Build history of the part. All positions in model axes, mm. A direction names the side the tool comes from. Give positions to 0.01 mm unless a question says otherwise; leave off trailing zeros. Loops run counter-clockwise (first coordinate to the right, second up) from the corner with the lowest first, then second, coordinate; pieces in that order, holes last.
1) Band-saw the part on B-B on z = 6.75. List the corners of the cut face in (x, y).
2) Wall check: line 1 (Y direction, x = 18.35, z = 4.25); line 2 (X direction, y = -12, z = 4); line 3 (X direction, y = -4.5, z = 3). Give the ranges that are in metal, low to high.
3) Flat gauge pins, fed straight in: P1, Ø1.1, axis at x = 24, y = 8, coming from the -Z side; P2, Ø1.1, axis at x = 26.5, y = 0, coming from the +Z side; P3, Ø4, axis at x = 26.5, z = 2.5, coming from the +Y side. Where does each tip first touch, or does it go through?
4) Two-plate mould, pull along Y, no slides. Class faces 1 (the flat face through (25, -9, 4)), 2 (the flat face through (25, -3, 6.15)): +Y half, -Y half, draft (parallel to the pull), parting line (faces both ways), or undercut.
5) 3-axis set-ups, long thin cutter, end or side, ignore diameter. For faces 3 (the cylindrical face through (-25.05, -12.44, 3.11)), 4 (the cylindrical face through (17.05, -12.04, 3.7)), 5 (the flat face through (25, -6.833, 4)), 6 (the flat face through (25, 8, 6.15)), 7 (the flat face through (0, 0, 0)): which of +Z, -Z, +X, -X, +Y, -Y reach the whole face in a straight line?
6) Band-saw the part on C-C on z = 3.65. State how many separate pieces and enclosed holes the cut face has, then the cut area to 3 significant figures.
7) Band-saw the part on A-A on x = 18.35. List the corners of the cut face in (y, z).
```python
from build123d import *

# Parameters (mm, degrees)
SKETCH1_W           = 42.5
SKETCH1_H           = 30
BOSS_EXTRUDE1_DEPTH = 7.3
CUT_EXTRUDE1_REACH  = 9.3
SKETCH2_R           = 1.3
SKETCH3_R           = 2.5
BOSS_EXTRUDE2_DEPTH = 7.7
SKETCH4_W           = 5
SKETCH4_H           = 1
BOSS_EXTRUDE3_DEPTH = 7.5


with BuildPart() as part:
    # Sketch1 → Boss-Extrude1 (new body)
    with BuildSketch(Plane.XY):
        Rectangle(SKETCH1_W, SKETCH1_H)
    extrude(amount=BOSS_EXTRUDE1_DEPTH)

    # Sketch2 → Cut-Extrude1 (cut, up to next)
    with BuildSketch(Plane.XY.offset(7.3), mode=Mode.PRIVATE) as cut_extrude1_sk1:
        with Locations((18.35, -12.1)):
            Circle(SKETCH2_R)
    cut_extrude1_tool1 = extrude(cut_extrude1_sk1.sketch, amount=-CUT_EXTRUDE1_REACH, mode=Mode.PRIVATE) & part.part
    add(cut_extrude1_tool1.solids().sort_by_distance((18.35, -12.1, 7.3))[0], mode=Mode.SUBTRACT)
    # Sketch2 → Cut-Extrude1 (cut, up to next)
    with BuildSketch(Plane.XY.offset(7.3), mode=Mode.PRIVATE) as cut_extrude1_sk2:
        with Locations((18.35, 12.1)):
            Circle(SKETCH2_R)
    cut_extrude1_tool2 = extrude(cut_extrude1_sk2.sketch, amount=-CUT_EXTRUDE1_REACH, mode=Mode.PRIVATE) & part.part
    add(cut_extrude1_tool2.solids().sort_by_distance((18.35, 12.1, 7.3))[0], mode=Mode.SUBTRACT)
    # Sketch2 → Cut-Extrude1 (cut, up to next)
    with BuildSketch(Plane.XY.offset(7.3), mode=Mode.PRIVATE) as cut_extrude1_sk3:
        with Locations((-18.95, 0)):
            Circle(SKETCH2_R)
    cut_extrude1_tool3 = extrude(cut_extrude1_sk3.sketch, amount=-CUT_EXTRUDE1_REACH, mode=Mode.PRIVATE) & part.part
    add(cut_extrude1_tool3.solids().sort_by_distance((-18.95, 0, 7.3))[0], mode=Mode.SUBTRACT)

    # Sketch3 → Boss-Extrude2 (add)
    with BuildSketch(Plane.ZY.offset(21.25)):
        with Locations((3.65, 10)):
            Circle(SKETCH3_R)
        with Locations((3.65, -10)):
            Circle(SKETCH3_R)
    extrude(amount=BOSS_EXTRUDE2_DEPTH)

    # Sketch4 → Boss-Extrude3 (add)
    with BuildSketch(Plane(origin=(21.25, 0, 0), x_dir=(0, 0, -1), z_dir=(1, 0, 0))):
        with Locations((-3.65, 9.5)):
            Rectangle(SKETCH4_W, SKETCH4_H)
        with Locations((-3.65, 7.916666667)):
            Rectangle(SKETCH4_W, SKETCH4_H)
        with Locations((-3.65, 6.333333333)):
            Rectangle(SKETCH4_W, SKETCH4_H)
        with Locations((-3.65, 4.75)):
            Rectangle(SKETCH4_W, SKETCH4_H)
        with Locations((-3.65, 3.166666667)):
            Rectangle(SKETCH4_W, SKETCH4_H)
        with Locations((-3.65, 1.583333333)):
            Rectangle(SKETCH4_W, SKETCH4_H)
        with Locations((-3.65, 0)):
            Rectangle(SKETCH4_W, SKETCH4_H)
        with Locations((-3.65, -1.583333333)):
            Rectangle(SKETCH4_W, SKETCH4_H)
        with Locations((-3.65, -3.166666667)):
            Rectangle(SKETCH4_W, SKETCH4_H)
        with Locations((-3.65, -4.75)):
            Rectangle(SKETCH4_W, SKETCH4_H)
        with Locations((-3.65, -6.333333333)):
            Rectangle(SKETCH4_W, SKETCH4_H)
        with Locations((-3.65, -7.916666667)):
            Rectangle(SKETCH4_W, SKETCH4_H)
        with Locations((-3.65, -9.5)):
            Rectangle(SKETCH4_W, SKETCH4_H)
    extrude(amount=BOSS_EXTRUDE3_DEPTH)


solid = part.part
```
Findings below:
1. outline: (-21.25, -15) - (21.25, -15) - (21.25, 15) - (-21.25, 15) - close; hole circle Ø2.6 at (-18.95, 0); hole circle Ø2.6 at (18.35, -12.1); hole circle Ø2.6 at (18.35, 12.1)
2. line 1: y = -15 to -13.4, -10.8 to 10.8, 13.4 to 15
2. line 2: x = -28.95 to 17.05, 19.65 to 21.25
2. line 3: x = -21.25 to 28.75
3. P1: stops at z = 1.15
3. P2: stops at z = 6.15
3. P3: stops at y = 10
4. face 1: undercut
4. face 2: draft
5. face 3: -X
5. face 4: +Z, -Z
5. face 5: +Z, -Z, +X
5. face 6: +Z, +X, +Y, -Y
5. face 7: -Z, +X, -X, +Y, -Y
6. separate pieces: 1
6. enclosed holes: 3
6. area: 1,430 mm2
7. outline: (-15, 0) - (-13.4, 0) - (-13.4, 7.3) - (-15, 7.3) - close; (-10.8, 0) - (10.8, 0) - (10.8, 7.3) - (-10.8, 7.3) - close; (13.4, 0) - (15, 0) - (15, 7.3) - (13.4, 7.3) - close
